from build123d import *

# Parameters (mm, degrees)
F0_R     = 1.25
F0_R_2   = 5
F1_DEPTH = 7
F2_R     = 1.5
F3_DEPTH = 46
F4_R     = 1.5
F5_DEPTH = 46


with BuildPart() as f1:
    # F0 (on Top) → F1 (new body)
    with BuildSketch(Plane.XY):
        Polygon((-23, -25.8675134595), (-20, -28.8675134595), (-10, -28.8675134595), (-10, -18.8675134595), (10, -18.8675134595), (10, -28.8675134595), (20, -28.8675134595), (20, -18.8675134595), (20, -11.5470053838), (26.3397459622, -7.8867513459), (30.4378221735, -8.9848275573), (33.9019237886, -6.9848275573), (35, -2.8867513459), (30, 5.7735026919), (21.3397459622, 0.7735026919), (11.3397459622, 18.0940107676), (20, 23.0940107676), (15, 31.7542648054), (10.9019237886, 32.8523410168), (7.4378221735, 30.8523410168), (6.3397459622, 26.7542648054), (0, 23.0940107676), (-6.3397459622, 26.7542648054), (-7.4378221735, 30.8523410168), (-10.9019237886, 32.8523410168), (-15, 31.7542648054), (-20, 23.0940107676), (-11.3397459622, 18.0940107676), (-21.3397459622, 0.7735026919), (-30, 5.7735026919), (-35, -2.8867513459), (-33.9019237886, -6.9848275573), (-30.4378221735, -8.9848275573), (-26.3397459622, -7.8867513459), (-20, -11.5470053838), (-20, -18.8675134595), (-23, -21.8675134595), align=None)
        with Locations((-10.8253175473, -6.25)):
            Circle(F0_R, mode=Mode.SUBTRACT)
        with Locations((0, -12.5)):
            Circle(F0_R, mode=Mode.SUBTRACT)
        with Locations((10.8253175473, -6.25)):
            Circle(F0_R, mode=Mode.SUBTRACT)
        Circle(F0_R_2, mode=Mode.SUBTRACT)
        with Locations((-10.8253175473, 6.25)):
            Circle(F0_R, mode=Mode.SUBTRACT)
        with Locations((10.8253175473, 6.25)):
            Circle(F0_R, mode=Mode.SUBTRACT)
        with Locations((0, 12.5)):
            Circle(F0_R, mode=Mode.SUBTRACT)
        Polygon((23, -21.8675134595), (23, -25.8675134595), (25, -23.8675134595), align=None)
        Polygon((20, -18.8675134595), (20, -28.8675134595), (23, -25.8675134595), (23, -21.8675134595), align=None)
    extrude(amount=F1_DEPTH)

    # F2 (on face) → F3 (cut)
    with BuildSketch(Plane(origin=(-11.5, -19.918584287, 0), x_dir=(0.8660254038, -0.5, 0), z_dir=(-0.5, -0.8660254038, 0))):
        with Locations((-23.8675134595, 3.5)):
            Circle(F2_R)
    extrude(amount=-F3_DEPTH, mode=Mode.SUBTRACT)

    # F4 (on face) → F5 (cut)
    with BuildSketch(Plane(origin=(-11.5, 19.918584287, 0), x_dir=(-0.8660254038, -0.5, 0), z_dir=(-0.5, 0.8660254038, 0))):
        with Locations((-23.8675134595, 3.5)):
            Circle(F4_R)
    extrude(amount=-F5_DEPTH, mode=Mode.SUBTRACT)


solid = f1.part
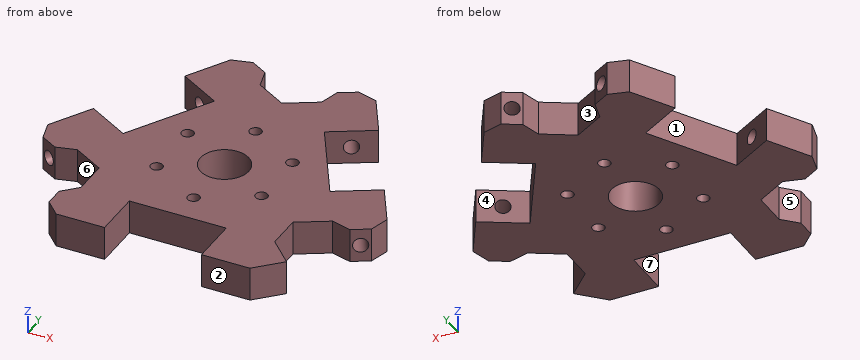
The listing builds one solid part. Answer for the finished solid, in the listing's coordinates (mm). Face numbers are marked on the shaded views. A direction names the side the tool comes from. Coordinates: 2 decimals unless noted, no trailing zeros. Write each loop counter-clockwise with the first axis right and the second up, starting at its lowest first coordinate (ties: lowest second). Pieces come first, ordered by that corner, then holes. Notation, with made-up numbers: M -40,85.25 L 16,85.25 A12 cw 16,97.25 Z; hole C 86.5,32 d4. An arc over 180 degrees is marked long. Put each result on its own line as item: value. Start each with the question number.
1. Flat-ended cylindrical pins translate along their axes: P1, Ø2, axis at y = -16, z = 4.5, coming from the +X side; P2, Ø2, axis at y = -25, z = 2.5, coming from the -X side; P3, Ø2, axis at x = 1, z = 2, coming from the -Y side. Find the tip coordinate at first contact, or state that the pin passes through.
2. A cutting plane is placed at C-C on z = 1.25. Count the separate pieces of the cut face and the enclosed holes in it, then the cut area to 3 significant figures.
3. Which of the six approach directions +Z, -Z, +X, -X, +Y, -Y give full straight-line access (tool end or side, diameter ignored) to the marked faces 4, 5, 6 and 7?
4. A cutting plane is placed at B-B on x = -2. Write down the section's boundary in (y, z).
5. A cutting plane is placed at A-A on y = -12.5. Write down the section's boundary in (x, z).
6. Consider line 1 (Y direction, x = 0, z = 2.5); line 2 (X direction, y = 1, z = 5.25); line 3 (X direction, y = -3, z = 5.25). Determine where each line is inside the solid, lowest interval first. Write a range as from..to.
7. For a pull along Y with two mould halves and no side action, classify the marked faces 1, 2 and 3 as pulls with the +Y half, pulls with the -Y half, needs draft (parallel to the pull), parting line crosses it, or undercut.
Resolved:
1. P1: stops at x = 20
1. P2: stops at x = -23
1. P3: stops at y = -18.87
2. separate pieces: 1
2. enclosed holes: 7
2. area: 2,190 mm2
3. face 4: +Z, -Z, +Y
3. face 5: +Z, -Z, -X
3. face 6: +Z, -Z
3. face 7: +Z, -Z, -Y
4. outline: M -18.87,0 L -4.58,0 L -4.58,7 L -18.87,7 Z; M 4.58,0 L 24.25,0 L 24.25,7 L 4.58,7 Z
5. outline: M -20,0 L -1.25,0 L -1.25,7 L -20,7 Z; M 1.25,0 L 20,0 L 20,7 L 1.25,7 Z
6. line 1: y = -18.87..-13.75, -11.25..-5, 5..11.25, 13.75..23.09
6. line 2: x = -32.76..-21.73, -21.21..-4.9, 4.9..21.21, 21.73..32.76
6. line 3: x = -34.97..-4, 4..34.97
7. face 1: undercut
7. face 2: pulls with the -Y half
7. face 3: pulls with the +Y half
